Verification items for the finished model (mm, model axes). A direction names the side the tool comes from. Round coordinates to 2 decimals unless told otherwise and drop trailing zeros. Return JSON: item names as keys, results as strings. Group by question number.
1) Tool access check on faces 1 (the flat face through (-906.5, 428.2, -493)), 2 (the flat face through (-4.867, 403.079, -34.808)). Record the directions out of +Z, -Z, +X, -X, +Y, -Y that give a thin tool (end or side, any length) a straight path to the whole face; none if there is none.
2) Depth check by flat-ended pin: pin 1 (1 mm diameter, centred on y = 515.5, z = -366, fed in from +X); pin 2 (1 mm diameter, centred on y = 493, z = -421.5, fed in from +X); pin 3 (3 mm diameter, centred on x = -757, z = -890.5, fed in from -Y). Enter the tip coordinate at first touch or a pass-through.
3) Draft check along X on faces 3 (the flat face through (-4.867, 403.079, -965.192)), 4 (the flat face through (-439, 417, 0)), 5 (the flat face through (37.724, 472.664, -493)). Enter one of: pulls with the +X half, pulls with the -X half, needs draft (parallel to the pull), parting line crosses it, or undercut.
4) Scan lines: L1, parallel to Y at x = -579, z = -272.5; L2, parallel to Y at x = -413.5, z = -921; L3, parallel to X at y = 446, z = -170.5. Record each from-to range of solid material in increasing order.
```python
from build123d import *


with BuildPart() as part:
    # Sweep1: sweep along a path in Sketch1
    with BuildLine(Plane.XY) as sweep1_path:
        ThreePointArc((-890.285718, 339.546922), (-431.638177, 392.054842), (29.914282, 382.890989))
    # Sketch3 → Sweep1 (sweep)
    with BuildSketch(Plane(origin=(-890.285718, 339.546922, 0), x_dir=(0, 0, 1), z_dir=(-0.983681, -0.179923, 0))):
        with BuildLine():
            Line((0, 0), (0, 60))
            ThreePointArc((0, 60), (-500, 145.786438), (-1000, 60))
            Line((-1000, 60), (-1000, 0))
            ThreePointArc((-1000, 0), (-500, 73.913317), (0, 0))
        make_face()
    sweep(path=sweep1_path.line)

    # Cut-Sweep1: sweep along a path in Sketch19
    with BuildLine(Plane(origin=(-205.375388, 17.865632, 0), x_dir=(0, 0, -1), z_dir=(0.996238, -0.086663, 0))) as cut_sweep1_path:
        ThreePointArc((70, 403.60426), (34.897149, 394.191626), (0, 384.042894))
    # Sketch4 → Cut-Sweep1 (sweep, cut)
    with BuildSketch(Plane.XY):
        with BuildLine():
            Line((-185.86158, 409.845466), (-187.161523, 394.901901))
            ThreePointArc((-187.161523, 394.901901), (-172.395032, 385.472889), (-157.121749, 394.056733))
            Line((-157.121749, 394.056733), (-155.821806, 409.000299))
            ThreePointArc((-155.821806, 409.000299), (-170.840774, 409.455574), (-185.86158, 409.845466))
        make_face()
    cut_sweep1 = sweep(path=cut_sweep1_path.line, mode=Mode.SUBTRACT)

    # Cut-Sweep6: sweep along a path in Sketch24
    with BuildLine(Plane(origin=(-54.770437, 4.764487, 0), x_dir=(0, 0, -1), z_dir=(0.996238, -0.086663, 0))) as cut_sweep6_path:
        ThreePointArc((70, 403.60426), (34.897149, 394.191626), (0, 384.042894))
    # Sketch22 → Cut-Sweep6 (sweep, cut)
    with BuildSketch(Plane.XY):
        with BuildLine():
            Line((-6.365403, 385.85431), (-5.10418, 400.352779))
            Line((-5.10418, 400.352779), (-34.991311, 402.952665))
            Line((-34.991311, 402.952665), (-36.291253, 388.009099))
            ThreePointArc((-36.291253, 388.009099), (-21.81537, 380.167646), (-6.365403, 385.85431))
        make_face()
    cut_sweep6 = sweep(path=cut_sweep6_path.line, mode=Mode.SUBTRACT)

    # Mirror1: Cut-Sweep1, Cut-Sweep6 across plane
    add(cut_sweep1.mirror(Plane.XY.offset(-500)), mode=Mode.SUBTRACT)
    add(cut_sweep6.mirror(Plane.XY.offset(-500)), mode=Mode.SUBTRACT)


solid = part.part
```
Check result:
{
 "1": {"face 1": "+Z, -Z, -X, -Y", "face 2": "none"},
 "2": {"pin 1": "x = 41.49", "pin 2": "x = 39.54", "pin 3": "y = 390.34"},
 "3": {"face 3": "undercut", "face 4": "needs draft", "face 5": "pulls with the +X half"},
 "4": {"L1": "441.06 to 510.89", "L2": "414.73 to 478.43", "L3": "-909.76 to 35.4"}
}
